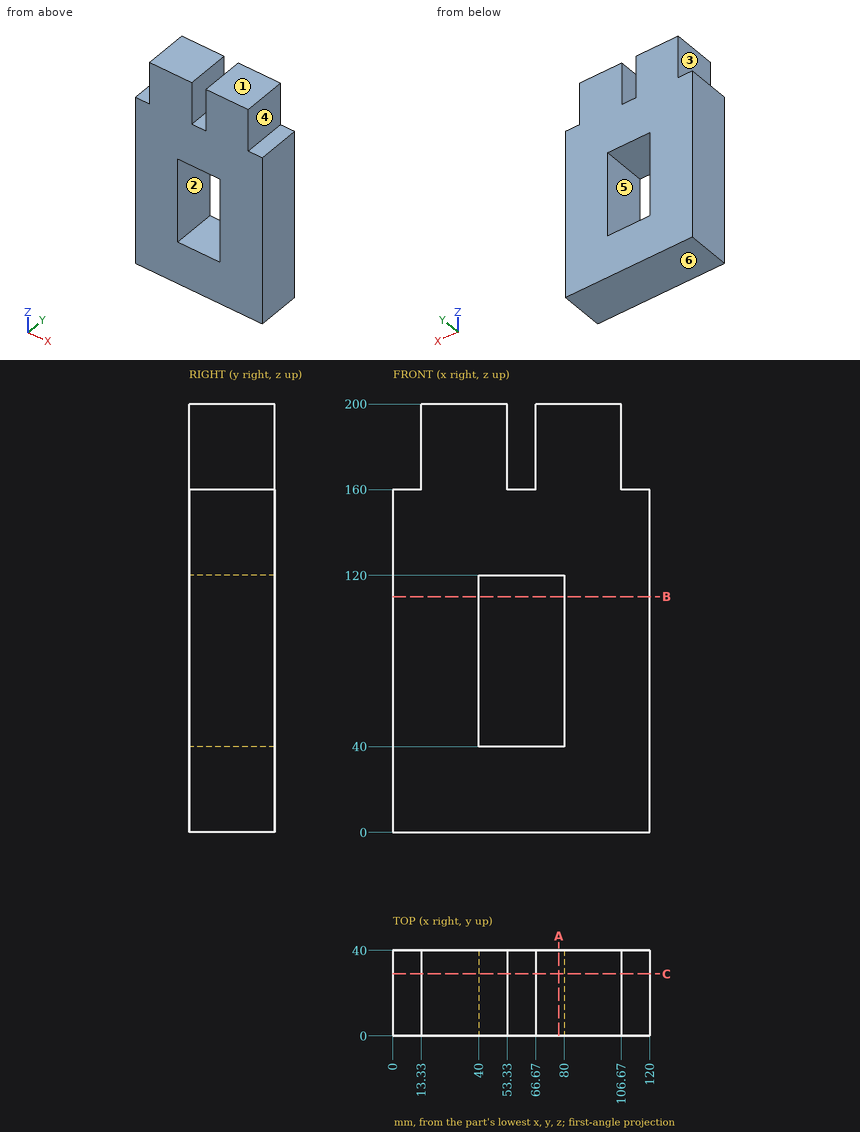
Job drawing, mm, ordinate dimensions from the low corner. One solid piece. A direction names the side the tool comes from. Coordinates: 2 decimals unless noted, no trailing zeros. Order: outer loops, then holes, each group sorted by start corner. A loop starts at its lowest first (then second) coordinate and runs counter-clockwise, first axis right, second up. Notation, with made-up numbers: (71, -27.75) - (128, -27.75) arc R8 ccw to (128, -21.75) - close; hole circle Ø3 at (-16, 20.25). An arc over 180 degrees is marked (long way). Write each question's results on one line, items separated by ' | '. Start each with the question number.
Item 1: Tool access for the marked faces 1 and 2: list every direction of +Z, -Z, +X, -X, +Y, -Y with a clear straight run to the whole face (end or side of a thin tool).
Item 2: Band-saw the part on B-B on z = 110. Write the cut outline in (x, y), and give its area (3 significant figures).
Item 3: Band-saw the part on A-A on x = 77.5. Write the cut outline in (y, z), and give its area (3 significant figures).
Item 4: Mould opens along X. For the marked faces 3, 4, 5 and 6 say: released by +X, released by -X, zero draft, split by the parting line, or undercut.
Item 5: Wall check: probe 1 along X at (y, z) = (11.5, 56); probe 2 along Z at (x, y) = (75.5, 23); probe 3 along X at (y, z) = (15, 165). Give the ranges that are in metal, low to high. Write a range as [from, to].
Item 6: Band-saw the part on C-C on y = 29. Write the cut outline in (x, z), and give its area (3 significant figures).
Item 7: Flat gauge pins, fed straight in: pin 1 (6 mm diameter, centred on x = 25, y = 10.5, fed in from -Z); pin 2 (12 mm diameter, centred on y = 13.5, z = 171, fed in from +X); pin 3 (6.5 mm diameter, centred on x = 113.5, y = 20.5, fed in from +Z); pin 4 (20 mm diameter, centred on y = 29.5, z = 181, fed in from -X). Where does each tip first touch, or does it go through?
Numbers:
1) face 1: +Z, +X, -X, +Y, -Y | face 2: +Y, -Y
2) outline: (0, 0) - (40, 0) - (40, 40) - (0, 40) - close; (80, 0) - (120, 0) - (120, 40) - (80, 40) - close | area: 3,200 mm^2
3) outline: (0, 0) - (40, 0) - (40, 40) - (0, 40) - close; (0, 120) - (40, 120) - (40, 200) - (0, 200) - close | area: 4,800 mm^2
4) face 3: released by -X | face 4: released by +X | face 5: undercut | face 6: zero draft
5) probe 1: [0, 40], [80, 120] | probe 2: [0, 40], [120, 200] | probe 3: [13.33, 53.33], [66.67, 106.67]
6) outline: (0, 0) - (120, 0) - (120, 160) - (106.67, 160) - (106.67, 200) - (66.67, 200) - (66.67, 160) - (53.33, 160) - (53.33, 200) - (13.33, 200) - (13.33, 160) - (0, 160) - close; hole (40, 40) - (80, 40) - (80, 120) - (40, 120) - close | area: 19,200 mm^2
7) pin 1: z = 0 | pin 2: x = 106.67 | pin 3: z = 160 | pin 4: x = 13.33
